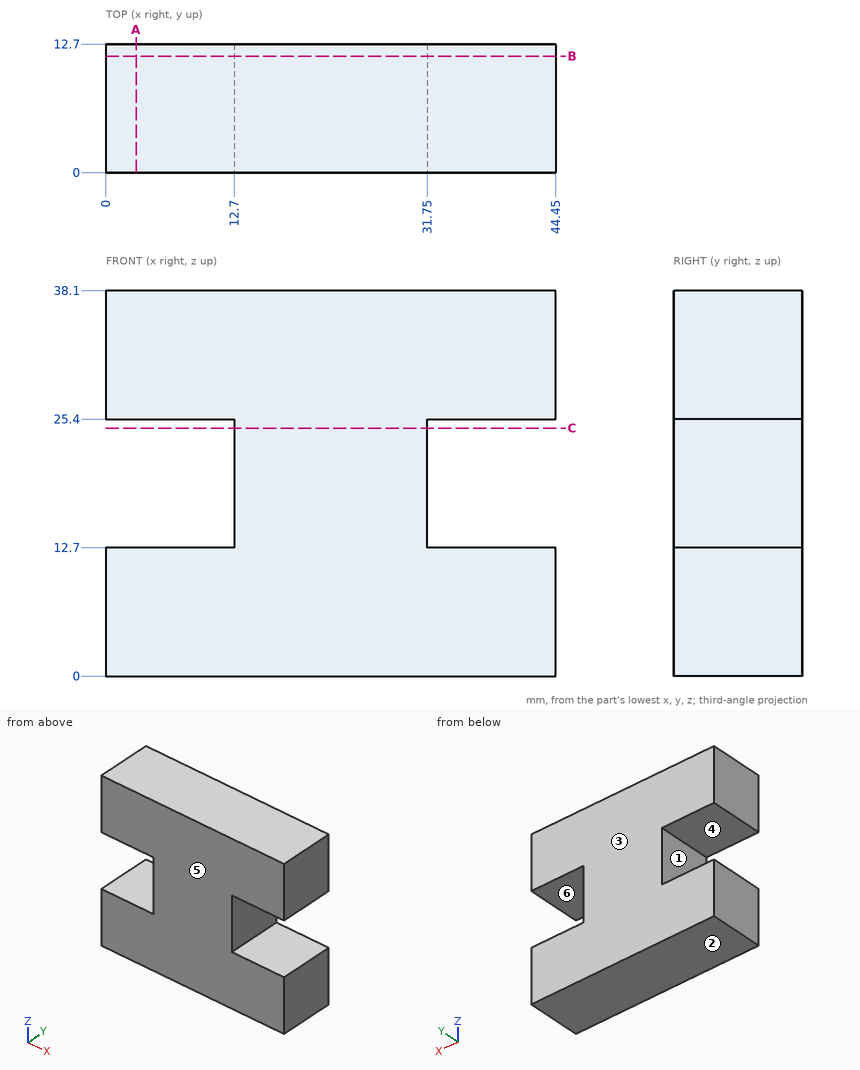
Study the drawing (mm; zero at the part's minimum x, y, z) and answer. A direction names the side the tool comes from. Give positions to 0.01 mm unless a question says otherwise; leave off trailing zeros. Order: outer loops, then holes, each group sorted by start corner. A loop starts at its lowest first (then second) coordinate and runs counter-clockwise, first axis right, second up. Notation, with made-up numbers: (79, 64) - (104, 64) arc R21 ccw to (104, 91) - close; hole circle Ø3 at (-13, 75). An arc over 180 degrees is marked (long way). Answer in a Markdown table with one row per item. Add a question column.
Q1. The part is cut by section A-A (x = 3). Determine the outline of the cut face in (y, z).
Q2. Which of the six approach directions +Z, -Z, +X, -X, +Y, -Y give full straight-line access (tool end or side, diameter ignored) to the marked faces 4, 5 and 6?
Q3. Find the intervals of material crossed by line 1 along Z through (x, y) = (38, 9.25); line 2 along X through (y, z) = (4.75, 15), in increasing order. Write a range as [from, to].
Q4. Given P1, Ø1, axis at y = 2, z = 20, coming from the -X side; P2, Ø6.5, axis at y = 7, z = 18.5, coming from the +X side, each flat-ended and moving along its own axis, determine where each tip first touches the part or whether it passes through.
Q5. For a pull along Z with two mould halves and no side action, classify the marked faces 1, 2 and 3 as released by +Z, released by -Z, zero draft, split by the parting line, or undercut.
Q6. The part is cut by section C-C (z = 24.5). Determine the outline of the cut face in (x, y), then the cut area to 3 significant figures.
Q7. The part is cut by section B-B (y = 11.5). Determine the outline of the cut face in (x, z).
Determined:
| question | item | result |
|---|---|---|
| 1 | outline | (0, 0) - (12.7, 0) - (12.7, 12.7) - (0, 12.7) - close; (0, 25.4) - (12.7, 25.4) - (12.7, 38.1) - (0, 38.1) - close |
| 2 | face 4 | -X, +Y, -Y |
| 2 | face 5 | +Z, -Z, +X, -X, -Y |
| 2 | face 6 | +X, +Y, -Y |
| 3 | line 1 | z = [0, 12.7], [25.4, 38.1] |
| 3 | line 2 | x = [12.7, 31.75] |
| 4 | P1 | stops at x = 12.7 |
| 4 | P2 | stops at x = 31.75 |
| 5 | face 1 | undercut |
| 5 | face 2 | released by -Z |
| 5 | face 3 | zero draft |
| 6 | outline | (12.7, 0) - (31.75, 0) - (31.75, 12.7) - (12.7, 12.7) - close |
| 6 | area | 242 mm² |
| 7 | outline | (0, 0) - (44.45, 0) - (44.45, 12.7) - (31.75, 12.7) - (31.75, 25.4) - (44.45, 25.4) - (44.45, 38.1) - (0, 38.1) - (0, 25.4) - (12.7, 25.4) - (12.7, 12.7) - (0, 12.7) - close |
